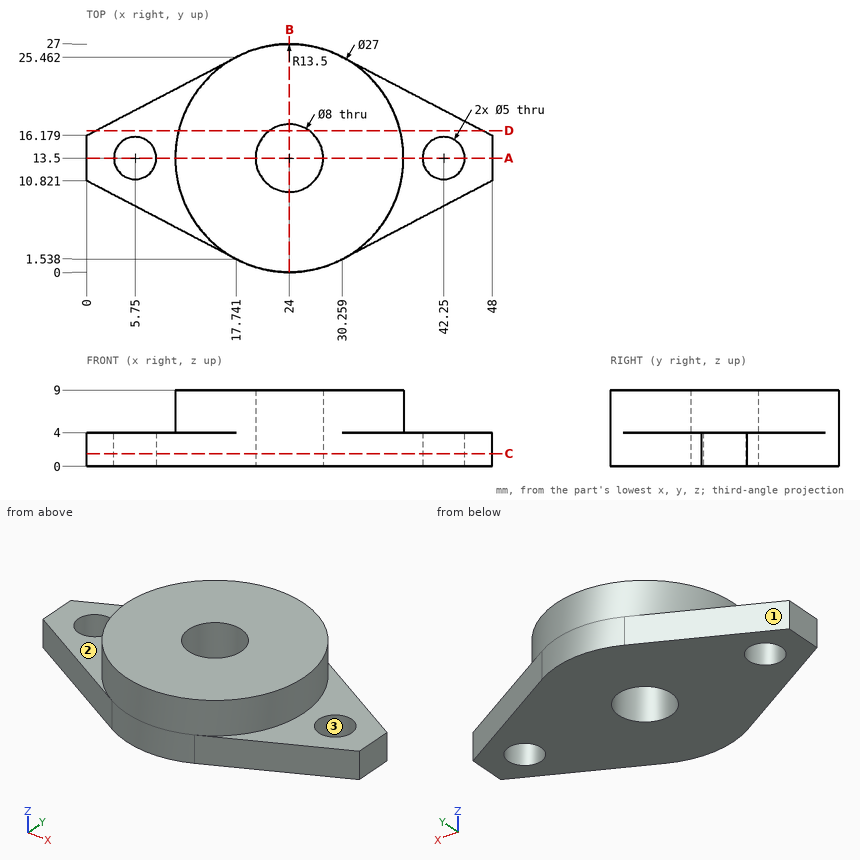
Design review of the part shown in the three views and the two pictorial views. Dimensions are in mm from the part's minimum x, y and z. Round coordinates to 2 decimals unless told otherwise and drop trailing zeros. Loops run counter-clockwise (first coordinate to the right, second up) from the corner with the lowest first, then second, coordinate; pieces in that order, holes last. Notation, with made-up numbers: M -6.75,21.5 L -1.75,21.5 A15 cw -1.75,35.5 Z; hole C 80.5,-19 d10. An arc over 180 degrees is marked long. Answer as a JSON object with one key per item and string values.
Item 1: We need section B-B on x = 24. Give the boundary of the cut face in (y, z), and give its area (3 significant figures).
Answer sheet:
{"outline": "M 0,0 L 9.5,0 L 9.5,9 L 0,9 Z; M 17.5,0 L 27,0 L 27,9 L 17.5,9 Z", "area": "171 mm^2"}
Item 2: We need section A-A on y = 13.5. Give the boundary of the cut face in (x, z), and give its area (3 significant figures).
Answer sheet:
{"outline": "M 0,0 L 3.25,0 L 3.25,4 L 0,4 Z; M 8.25,0 L 20,0 L 20,9 L 10.5,9 L 10.5,4 L 8.25,4 Z; M 28,0 L 39.75,0 L 39.75,4 L 37.5,4 L 37.5,9 L 28,9 Z; M 44.75,0 L 48,0 L 48,4 L 44.75,4 Z", "area": "215 mm^2"}
Item 3: We need section C-C on z = 1.5. Give the boundary of the cut face in (x, y).
Answer sheet:
{"outline": "M 0,10.82 L 17.74,1.54 A13.5 ccw 30.26,1.54 L 48,10.82 L 48,16.18 L 30.26,25.46 A13.5 ccw 17.74,25.46 L 0,16.18 Z; hole C 5.75,13.5 d5; hole C 24,13.5 d8; hole C 42.25,13.5 d5"}
Item 4: Wall thickness on L1, parallel to X at y = 14.75, z = 1.75 (1 decimal); L2, parallel to Y at x = 24, z = 6.5; L3, parallel to X at y = 13.75, z = 6: over which ranges is each line inside the solid? List them lowest first. Write a range as from..to.
Answer sheet:
{"L1": "x = 0..3.6, 7.9..20.2, 27.8..40.1, 44.4..48", "L2": "y = 0..9.5, 17.5..27", "L3": "x = 10.5..20.01, 27.99..37.5"}
Item 5: The part is to be moulded in two halves that separate along Y. For the marked faces 1, 2 and 3, say which applies: pulls with the +Y half, pulls with the -Y half, needs draft (parallel to the pull), parting line crosses it, or undercut.
Answer sheet:
{"face 1": "pulls with the +Y half", "face 2": "needs draft", "face 3": "undercut"}
Item 6: Clearance check with flat-ended pins moving along their axes: P1, Ø14, axis at x = 38, y = 14.5, coming from the +Z side; P2, Ø4, axis at x = 5.75, y = 13.5, coming from the +Z side; P3, Ø5, axis at y = 22.5, z = 7.5, coming from the +X side. State where each tip first meets the part, or that it passes through.
Answer sheet:
{"P1": "stops at z = 9", "P2": "passes through", "P3": "stops at x = 35.83"}
Item 7: We need section D-D on y = 16.75. Give the boundary of the cut face in (x, z).
Answer sheet:
{"outline": "M 1.09,0 L 21.67,0 L 21.67,9 L 10.9,9 L 10.9,4 L 1.09,4 Z; M 26.33,0 L 46.91,0 L 46.91,4 L 37.1,4 L 37.1,9 L 26.33,9 Z"}
